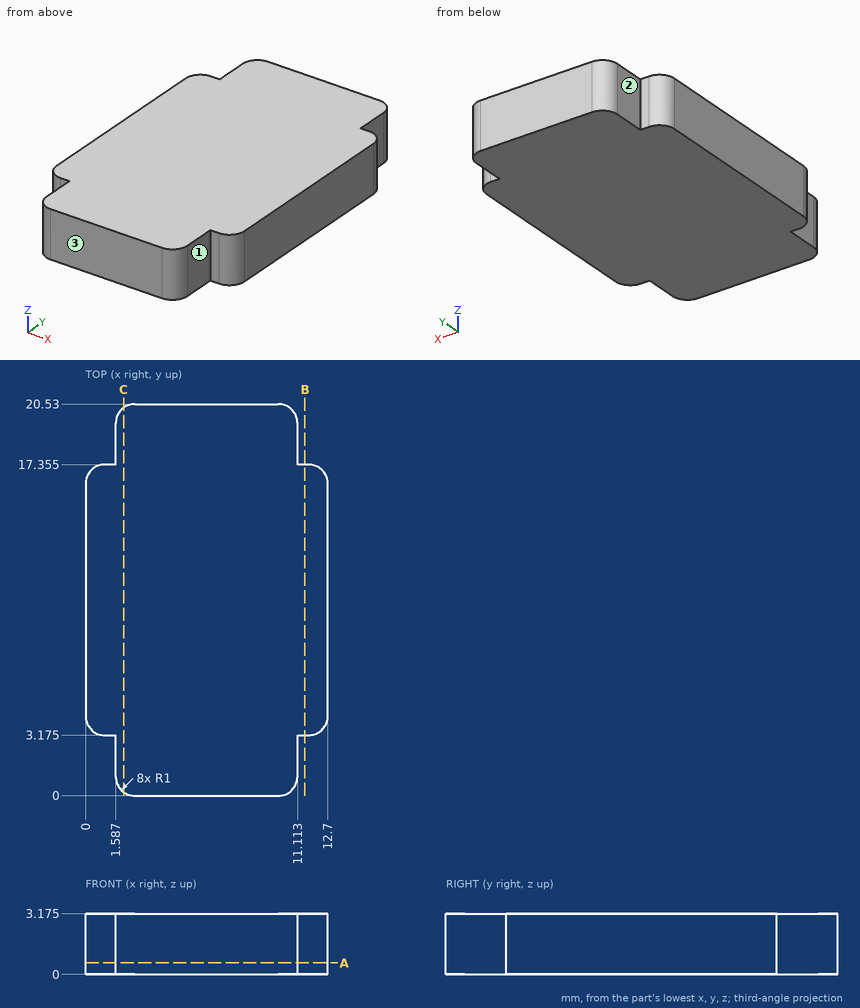
Input: dimensioned drawing with shaded views. Units: mm. Origin: part minimum x, y, z. A direction names the side the tool comes from. Round coordinates to 2 decimals unless told otherwise and drop trailing zeros. Order: outer loops, then holes, each group sorted by start corner. A loop starts at its lowest first (then second) coordinate and runs counter-clockwise, first axis right, second up. Notation, with made-up numbers: (85.5, 81) -> (127.5, 81) arc R9 cw to (127.5, 88) -> close; hole circle Ø5 at (39, -29). An arc over 180 degrees is marked (long way). One line per item, written item: value. Start each with the question number.
Q1. Section query B-B (x = 11.5). Return the cut outline in (y, z) (1 decimal).
Q2. Access query for the marked faces 1, 2 and 3. Directions: +Z, -Z, +X, -X, +Y, -Y. A direction counts if a zero-diameter tool reaches every point of the face in a straight line with its end or side. Return the directions, or none.
Q3. Pin query (flat end, axial travel): pin 1 (0.6 mm diameter, centred on x = 11.5, z = 1, fed in from -Y) (1 decimal); pin 2 (1.7 mm diameter, centred on y = 18.5, z = 1, fed in from +X); pin 3 (1.7 mm diameter, centred on y = 19, z = 1.5, fed in from -X). Return the tip coordinate at first contact, or that it passes through.
Q4. Material intervals for probe 1 along X at (y, z) = (2.75, 2.55); probe 2 along Y at (x, z) = (11.75, 2.65); probe 3 along Y at (x, z) = (12, 0.4), sorted ascending.
Q5. Section query C-C (x = 2). Return the cut outline in (y, z) (1 decimal).
Q6. Section query A-A (z = 0.6). Return the cut outline in (x, y) (1 decimal), plus the area to 3 significant figures.
Findings below:
1. outline: (3.2, 0) -> (17.4, 0) -> (17.4, 3.2) -> (3.2, 3.2) -> close
2. face 1: +Z, -Z, +X, -Y
2. face 2: +Z, -Z, -X, +Y
2. face 3: +Z, -Z, +X, -X, -Y
3. pin 1: y = 3.2
3. pin 2: x = 11.11
3. pin 3: x = 1.59
4. probe 1: 1.59 to 11.11
4. probe 2: 3.18 to 17.35
4. probe 3: 3.22 to 17.31
5. outline: (0.2, 0) -> (20.3, 0) -> (20.3, 3.2) -> (0.2, 3.2) -> close
6. outline: (0, 4.2) arc R1 ccw to (1, 3.2) -> (1.6, 3.2) -> (1.6, 1) arc R1 ccw to (2.6, 0) -> (10.1, 0) arc R1 ccw to (11.1, 1) -> (11.1, 3.2) -> (11.7, 3.2) arc R1 ccw to (12.7, 4.2) -> (12.7, 16.4) arc R1 ccw to (11.7, 17.4) -> (11.1, 17.4) -> (11.1, 19.5) arc R1 ccw to (10.1, 20.5) -> (2.6, 20.5) arc R1 ccw to (1.6, 19.5) -> (1.6, 17.4) -> (1, 17.4) arc R1 ccw to (0, 16.4) -> close
6. area: 239 mm²
